from build123d import *

# Parameters (mm, degrees)
SKETCH1_W                  = 76.2
SKETCH1_H                  = 25.4
EXTRUDE1_DEPTH             = 49.53
SKETCH2_W                  = 6.35
SKETCH2_H                  = 20.32
EXTRUDE2_DEPTH             = 95.36535858
FILLET1_R                  = 2.54
F_10_32_TAPPED_HOLE1_D     = 4.0386
F_10_32_TAPPED_HOLE1_DEPTH = 13.6144
F_10_32_TAPPED_HOLE1_TIP   = 1.213317848


with BuildPart() as part:
    # Sketch1 → Extrude1 (new body)
    with BuildSketch(Plane.XY):
        with Locations((38.1, 12.7)):
            Rectangle(SKETCH1_W, SKETCH1_H)
    extrude(amount=EXTRUDE1_DEPTH)

    # Sketch2 → Extrude2 (cut, through all)
    with BuildSketch(Plane.XZ):
        with Locations((57.260871328, 39.37)):
            Rectangle(SKETCH2_W, SKETCH2_H)
    extrude(amount=-EXTRUDE2_DEPTH, mode=Mode.SUBTRACT)

    # Fillet1
    fillet1_edges = [part.edges().sort_by_distance(p)[0] for p in [
        (76.2, 12.7, 49.53),
        (68.317935664, 25.4, 49.53),
        (68.317935664, 0, 49.53),
        (27.042935664, 25.4, 49.53),
        (0, 12.7, 49.53),
        (27.042935664, 0, 49.53),
        (0, 25.4, 24.765),
        (76.2, 25.4, 24.765),
        (76.2, 0, 24.765),
        (0, 0, 24.765),
    ]]
    fillet(fillet1_edges, radius=FILLET1_R)

    # #10-32 Tapped Hole1
    with Locations(Plane(origin=(66.04, 12.7, 0), x_dir=(-1, 0, 0), z_dir=(0, 0, -1))):
        with Locations((0, 0), (46.99, 0)):
            Hole(F_10_32_TAPPED_HOLE1_D / 2, depth=F_10_32_TAPPED_HOLE1_DEPTH)
            with Locations((0, 0, -(F_10_32_TAPPED_HOLE1_DEPTH + F_10_32_TAPPED_HOLE1_TIP / 2))):  # 118° drill point
                Cone(0, F_10_32_TAPPED_HOLE1_D / 2, F_10_32_TAPPED_HOLE1_TIP, mode=Mode.SUBTRACT)


solid = part.part
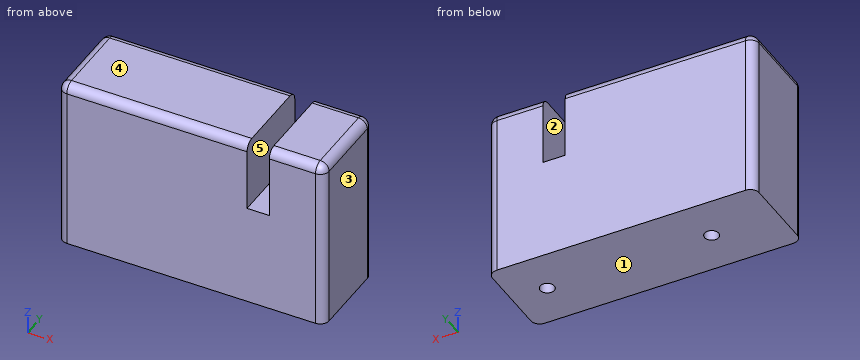
Build history of the part. All positions in model axes, mm. Face numbers are marked on the shaded views. A direction names the side the tool comes from. Coordinates: 2 decimals unless noted, no trailing zeros. Order: outer loops, then holes, each group sorted by start corner. A loop starts at its lowest first (then second) coordinate and runs counter-clockwise, first axis right, second up. Notation, with made-up numbers: (46, -25) -> (97, -25) arc R35 ccw to (97, 14) -> close; hole circle Ø8 at (-38.5, 18). An arc over 180 degrees is marked (long way). One line per item, written item: value.
(1) Slice it at C-C, the plane y = 22. List the corners of the cut face in (x, z), plus the area to 3 significant figures.
Checked values:
outline: (0, 0) -> (76.2, 0) -> (76.2, 46.99) arc R2.54 ccw to (73.66, 49.53) -> (60.44, 49.53) -> (60.44, 29.21) -> (54.09, 29.21) -> (54.09, 49.53) -> (2.54, 49.53) arc R2.54 ccw to (0, 46.99) -> close
area: 3,640 mm2
(2) Slice it at B-B, the plane z = 9. List the corners of the cut face in (x, y), plus the area to 3 significant figures.
Checked values:
outline: (0, 2.54) arc R2.54 ccw to (2.54, 0) -> (73.66, 0) arc R2.54 ccw to (76.2, 2.54) -> (76.2, 22.86) arc R2.54 ccw to (73.66, 25.4) -> (2.54, 25.4) arc R2.54 ccw to (0, 22.86) -> close; hole circle Ø4.04 at (19.05, 12.7); hole circle Ø4.04 at (66.04, 12.7)
area: 1,900 mm2
(3) Probe line 1 (X direction, y = 12.7, z = 10.75); line 2 (Y direction, x = 66, z = 4); line 3 (X direction, y = 7.5, z = 39.5). List the from-to ranges inside material, lowest first. Write a range as [from, to].
Checked values:
line 1: [0, 17.03], [21.07, 64.02], [68.06, 76.2]
line 2: [0, 10.68], [14.72, 25.4]
line 3: [0, 54.09], [60.44, 76.2]
(4) Tool access for the marked faces 4 and 5: list every direction of +Z, -Z, +X, -X, +Y, -Y with a clear straight run to the whole face (end or side of a thin tool).
Checked values:
face 4: +Z, +X, -X, +Y, -Y
face 5: +Z, +Y, -Y
(5) Slice it at A-A, the plane z = 44.5. List the corners of the cut face in (x, y).
Checked values:
outline: (0, 2.54) arc R2.54 ccw to (2.54, 0) -> (54.09, 0) -> (54.09, 25.4) -> (2.54, 25.4) arc R2.54 ccw to (0, 22.86) -> close; (60.44, 0) -> (73.66, 0) arc R2.54 ccw to (76.2, 2.54) -> (76.2, 22.86) arc R2.54 ccw to (73.66, 25.4) -> (60.44, 25.4) -> close
(6) Drop flat-ended pins along their axis: pin 1 Ø1.9 at (x, y) = (57.5, 7.5) entering from +Z; pin 2 Ø2.5 at (x, y) = (19.05, 12.7) entering from -Z. Give the stop position or say it passes through.
Checked values:
pin 1: z = 29.21
pin 2: z = 14.08
(7) Mould opens along X. For the marked faces 1, 2 and 3 say: pulls with the +X half, pulls with the -X half, needs draft (parallel to the pull), parting line crosses it, or undercut.
Checked values:
face 1: needs draft
face 2: undercut
face 3: pulls with the +X half
